```python
from build123d import *

# Parameters (mm, degrees)
F1_DEPTH = 50
F2_W     = 4
F2_H     = 30
F3_DEPTH = 25


with BuildPart() as f1:
    # F0 (on Front) → F1 (new body)
    with BuildSketch(Plane.XZ):
        Polygon((-10.624999, 12), (-40.624999, 12), (-40.624999, 4.5), (-37.624999, 4.5), (-37.624999, 8.751204), (-30.624999, 8.751204), (-30.624999, 1.751204), (-37.624999, 1.751204), (-37.624999, 2.7), (-40.624999, 2.7), (-40.624999, 0), (-10.624999, 0), align=None)
    extrude(amount=F1_DEPTH)

    # F2 (on face) → F3 (cut)
    with BuildSketch(Plane.XY.offset(12)):
        with Locations((-17.624999, -25)):
            Rectangle(F2_W, F2_H)
    extrude(amount=-F3_DEPTH, mode=Mode.SUBTRACT)


solid = f1.part
```
Geometry check sheet. Reference: the model listing, model coordinates, mm. A direction names the side the tool comes from. Coordinates: 2 decimals unless noted, no trailing zeros. Order: outer loops, then holes, each group sorted by start corner. A loop starts at its lowest first (then second) coordinate and runs counter-clockwise, first axis right, second up. Notation, with made-up numbers: (85.5, 71.25) - (105.5, 71.25) arc R24 cw to (105.5, 97.25) - close; hole circle Ø4 at (17, 45.5). An arc over 180 degrees is marked (long way). Answer in a Markdown table with one row per item. Add a question column.
1. Access from +Z, -Z, +X, -X, +Y, -Y to the whole of each face (thin tool, end or side, straight path). Record for faces 4 (the face through (-26, 0, 6)), 5 (the face through (-34, -25, 1.751)), 6 (the face through (-15.625, -25, 6)), 7 (the face through (-40.625, -25, 8)), 8 (the face through (-39, -25, 4.5)).
2. Draft check along Z on faces 1 (the face through (-26, -25, 0)), 2 (the face through (-39, -25, 2.7)), 3 (the face through (-26, -50, 6)). Enter one of: +Z half, -Z half, draft (parallel to the pull), parting line (faces both ways), or undercut.
3. Section check B-B (y = -34). Enter the section's corners in (x, z) (3 decimals), plus the area to 3 significant figures.
4. Section check C-C (x = -33.75). Enter the section's corners in (y, z), plus the area to 3 significant figures.
5. Section check D-D (z = 11). Enter the section's corners in (x, y) (3 decimals), plus the area to 3 significant figures.
6. Material ranges on L1, parallel to X at y = -23, z = 7.25 (3 decimals); L2, parallel to X at y = -37, z = 4 (3 decimals); L3, parallel to Z at x = -33.5, y = -31, recorded low to high. Write a range as [from, to].
7. Section check A-A (z = 5.75). Enter the section's corners in (x, y) (3 decimals), plus the area to 3 significant figures.
Data:
| question | item | result |
|---|---|---|
| 1 | face 4 | +Z, -Z, +X, -X, +Y |
| 1 | face 5 | +Y, -Y |
| 1 | face 6 | +Z, -Z |
| 1 | face 7 | +Z, -Z, -X, +Y, -Y |
| 1 | face 8 | -X, +Y, -Y |
| 2 | face 1 | -Z half |
| 2 | face 2 | undercut |
| 2 | face 3 | draft |
| 3 | outline | (-40.625, 0) - (-19.625, 0) - (-19.625, 12) - (-40.625, 12) - (-40.625, 4.5) - (-37.625, 4.5) - (-37.625, 8.751) - (-30.625, 8.751) - (-30.625, 1.751) - (-37.625, 1.751) - (-37.625, 2.7) - (-40.625, 2.7) - close; (-15.625, 0) - (-10.625, 0) - (-10.625, 12) - (-15.625, 12) - close |
| 3 | area | 258 mm² |
| 4 | outline | (-50, 0) - (0, 0) - (0, 1.75) - (-50, 1.75) - close; (-50, 8.75) - (0, 8.75) - (0, 12) - (-50, 12) - close |
| 4 | area | 250 mm² |
| 5 | outline | (-40.625, -50) - (-10.625, -50) - (-10.625, 0) - (-40.625, 0) - close; hole (-19.625, -40) - (-15.625, -40) - (-15.625, -10) - (-19.625, -10) - close |
| 5 | area | 1,380 mm² |
| 6 | L1 | x = [-40.625, -37.625], [-30.625, -19.625], [-15.625, -10.625] |
| 6 | L2 | x = [-30.625, -19.625], [-15.625, -10.625] |
| 6 | L3 | z = [0, 1.75], [8.75, 12] |
| 7 | outline | (-40.625, -50) - (-37.625, -50) - (-37.625, 0) - (-40.625, 0) - close; (-30.625, -50) - (-10.625, -50) - (-10.625, 0) - (-30.625, 0) - close; hole (-19.625, -40) - (-15.625, -40) - (-15.625, -10) - (-19.625, -10) - close |
| 7 | area | 1,030 mm² |
